Can you work these out from the model? Positions are in its coordinate system, mm. A direction names the side the tool comes from. Coordinates: 2 decimals unless noted, no trailing zeros. Loops run counter-clockwise (first coordinate to the right, second up) from the corner with the lowest first, then second, coordinate; pieces in that order, holes last.
Autodesk Inventor part; units mm, degrees
ref_plane "YZ Plane" through (0, 0, 0) normal (1, 0, 0) x (0, 1, 0)
ref_plane "XZ Plane" through (0, 0, 0) normal (0, 1, 0) x (-1, 0, 0)
ref_plane "XY Plane" through (0, 0, 0) normal (0, 0, 1) x (1, 0, 0)
sketch "Sketch1" plane through (0, 0, 0) normal (1, 0, 0) x (0, 1, 0)
  line L0 (0, 0) -> (20, 0)
  line L1 (20, 0) -> (20, -10)
  line L2 (20, -10) -> (0, -10)
  line L3 (0, -10) -> (0, 0)
  line L4 (20, -10) -> (50, -10)
  line L5 (50, -10) -> (50, 0)
  line L6 (50, 0) -> (20, 0)
  line L7 (20, 0) -> (20, -10)
  line L8 (50, 0) -> (40, 0)
  line L9 (40, 0) -> (40, -50)
  line L10 (40, -50) -> (50, -50)
  line L11 (50, -50) -> (50, 0)
  line L12 (40, -50) -> (50, -50)
  line L13 (50, -50) -> (50, -30)
  line L14 (50, -30) -> (40, -30)
  line L15 (40, -30) -> (40, -50)
  line L16 (20, -10) -> (40, -30)
  line L17 (40, -10) -> (20, -10)
  line L18 (40, -10) -> (40, -30)
  dimension "d0" = 20
  dimension "d1" = 10
  dimension "d2" = 30
  dimension "d3" = 10
  dimension "d4" = 10
  dimension "d5" = 50
  dimension "d6" = 10
  dimension "d7" = 20
extrude "Extrusion1" add sketch "Sketch1" along normal blind 20
sketch "Sketch2" plane through (0, 50, 0) normal (0, 1, 0) x (1, 0, 0)
  circle A0 centre (10, 40) radius 2.75
  line L0 (20, 50) -> (20, 0)
  line L1 (0, 50) -> (20, 50)
  point P0 (0, 0)
  dimension "d10" = 5.5
  dimension "d11" = 10
  dimension "d12" = 10
extrude "Extrusion2" cut sketch "Sketch2" against normal blind 20
sketch "Sketch3" plane through (0, 0, 0) normal (0, 0, 1) x (1, 0, 0)
  circle A0 centre (10, 10) radius 2.75
  line L0 (0, 0) -> (20, 0)
  line L1 (20, 50) -> (20, 0)
  dimension "d15" = 5.5
  dimension "d16" = 10
  dimension "d17" = 10
extrude "Extrusion3" cut sketch "Sketch3" against normal blind 20
properties part number "Standard Bracing" material "Aluminum 6061"
Item 1: I'm going to push flat-ended pins straight in: P1, Ø8, axis at x = 8, y = 43, coming from the +Z side; P2, Ø5, axis at x = 3, z = -26.5, coming from the -Y side; P3, Ø12, axis at x = 15, z = -34, coming from the -Y side; P4, Ø5, axis at x = 10, z = -40, coming from the -Y side. Where does each tip first touch, or does it pass through?
Results are:
P1: stops at z = 0
P2: stops at y = 34
P3: stops at y = 38
P4: passes through
Item 2: I need wall thicknesses on line 1 along Y through (x, z) = (10, -4.25); line 2 along Z through (x, y) = (10, 44.75); line 3 along Y through (x, z) = (15, -40). Which ranges of each line are inside material? Lowest first, please.
Results are:
line 1: y = 0 to 7.25, 12.75 to 50
line 2: z = -50 to -42.75, -37.25 to 0
line 3: y = 40 to 50
Item 3: Suppose I cut it at B-B, the plane y = 10. Please give me the cut outline in (x, z).
Results are:
outline: (0, -10) - (7.25, -10) - (7.25, 0) - (0, 0) - close; (12.75, -10) - (20, -10) - (20, 0) - (12.75, 0) - close
Item 4: Suppose I cut it at A-A, the plane x = 10. Please give me the cut outline in (y, z), plus the area to 3 significant figures.
Results are:
outline: (0, -10) - (7.25, -10) - (7.25, 0) - (0, 0) - close; (12.75, -10) - (20, -10) - (40, -30) - (40, -37.25) - (50, -37.25) - (50, 0) - (12.75, 0) - close; (40, -50) - (50, -50) - (50, -42.75) - (40, -42.75) - close
area: 990 mm2
Item 5: Suppose I cut it at D-D, the plane z = -9. Please give me the cut outline in (x, y), plus the area to 3 significant figures.
Results are:
outline: (0, 0) - (20, 0) - (20, 50) - (0, 50) - close; hole circle Ø5.5 at (10, 10)
area: 976 mm2
Item 6: We'd pull the mould along X, two halves only. Please class faces 3 (the face through (0, 36, -14)), 4 (the face through (7.6, 12.4, -10)), 5 (the face through (11.48, 12.32, -4.93)): +X half, -X half, draft (parallel to the pull), parting line (faces both ways), or undercut.
Results are:
face 3: -X half
face 4: draft
face 5: undercut
Item 7: Suppose I cut it at C-C, the plane z = -40. Please give me the cut outline in (x, y).
Results are:
outline: (0, 40) - (7.25, 40) - (7.25, 50) - (0, 50) - close; (12.75, 40) - (20, 40) - (20, 50) - (12.75, 50) - close
Item 8: On a 3-axis mill with a long thin cutter (end or side, diameter ignored), from which of +Z, -Z, +X, -X, +Y, -Y can I reach the whole of each face in a straight line? I mean faces 1 (the face through (7.6, 40, -37.6)), 2 (the face through (10, 50, -25)). Say none if no direction works.
Results are:
face 1: -Z, +X, -X, -Y
face 2: +Z, -Z, +X, -X, +Y
